Source: CAD feature listing. Evaluate the final solid. Frame: model axes, mm. A direction names the side the tool comes from. Give positions to 0.01 mm unless a question says otherwise; leave off trailing zeros. Order: outer loops, then holes, each group sorted by start corner. A loop starts at its lowest first (then second) coordinate and runs counter-clockwise, first axis right, second up.
```python
from build123d import *

# Parameters (mm, degrees)
BOSS_EXTRUDE1_DEPTH = 6.35
CUT_EXTRUDE1_DEPTH  = 212.713804804
SKETCH5_W           = 12.7
SKETCH5_H           = 30
CUT_EXTRUDE3_DEPTH  = 212.713804804


with BuildPart() as part:
    # Sketch2 → Boss-Extrude1 (new body)
    with BuildSketch(Plane(origin=(0, 0, 0), x_dir=(1, 0, 0), z_dir=(0, 1, 0))):
        with BuildLine():
            Line((-2.579558011, -38.687016575), (16.470441989, -38.687016575))
            Line((16.470441989, -38.687016575), (16.470441989, 20.312983425))
            Line((16.470441989, 20.312983425), (22.470441989, 20.312983425))
            ThreePointArc((22.470441989, 20.312983425), (23.17754877, 20.605876644), (23.470441989, 21.312983425))
            Line((23.470441989, 21.312983425), (23.470441989, 69.312983425))
            ThreePointArc((23.470441989, 69.312983425), (23.17754877, 70.020090207), (22.470441989, 70.312983425))
            Line((22.470441989, 70.312983425), (16.470441989, 70.312983425))
            Line((16.470441989, 70.312983425), (16.470441989, 130.312983425))
            Line((16.470441989, 130.312983425), (22.470441989, 130.312983425))
            ThreePointArc((22.470441989, 130.312983425), (23.17754877, 130.605876644), (23.470441989, 131.312983425))
            Line((23.470441989, 131.312983425), (23.470441989, 179.312983425))
            ThreePointArc((23.470441989, 179.312983425), (23.17754877, 180.020090207), (22.470441989, 180.312983425))
            Line((22.470441989, 180.312983425), (16.470441989, 180.312983425))
            Line((16.470441989, 180.312983425), (16.470441989, 210.312983425))
            Line((16.470441989, 210.312983425), (-2.579558011, 210.312983425))
            Line((-2.579558011, 210.312983425), (-2.579558011, -38.687016575))
        make_face()
    extrude(amount=BOSS_EXTRUDE1_DEPTH)

    # Sketch3 → Cut-Extrude1 (cut, through all)
    with BuildSketch(Plane(origin=(0, 6.35, 0), x_dir=(1, 0, 0), z_dir=(0, 1, 0))):
        with BuildLine():
            Line((16.470441989, 61.312983425), (4.470441989, 61.312983425))
            ThreePointArc((4.470441989, 61.312983425), (3.056228427, 61.898769863), (2.470441989, 63.312983425))
            Line((2.470441989, 63.312983425), (2.470441989, 89.312983425))
            ThreePointArc((2.470441989, 89.312983425), (3.056228427, 90.727196988), (4.470441989, 91.312983425))
            Line((4.470441989, 91.312983425), (16.470441989, 91.312983425))
            Line((16.470441989, 91.312983425), (16.470441989, 61.312983425))
        make_face()
    extrude(amount=-CUT_EXTRUDE1_DEPTH, mode=Mode.SUBTRACT)

    # Sketch5 → Cut-Extrude3 (cut, through all)
    with BuildSketch(Plane.XZ):
        with Locations((10.120441989, -116.312983425)):
            Rectangle(SKETCH5_W, SKETCH5_H)
    extrude(amount=-CUT_EXTRUDE3_DEPTH, mode=Mode.SUBTRACT)


solid = part.part
```
1) Draft query along Z for faces 4 (the flat face through (19, 3, -20.313)), 5 (the flat face through (16.47, 3, 10)), 6 (the flat face through (16.47, 3, -66)). Return one class per face: +Z half, -Z half, draft (parallel to the pull), parting line (faces both ways), or undercut.
Report:
face 4: +Z half
face 5: draft
face 6: undercut
2) Material intervals for L1, parallel to Z at x = 8.25, y = 2.5; L2, parallel to Z at x = 21.5, y = 3; L3, parallel to Z at x = 3.5, y = 5, sorted ascending.
Report:
L1: z = -210.31 to -131.31, -101.31 to -91.31, -61.31 to 38.69
L2: z = -180.31 to -130.31, -70.31 to -20.31
L3: z = -210.31 to -91.06, -61.56 to 38.69
3) Section query B-B, the plane y = 4.75. Return the cut outline in (x, z), and give its area (3 significant figures).
Report:
outline: (-2.58, -210.31) - (16.47, -210.31) - (16.47, -180.31) - (22.47, -180.31) arc R1 ccw to (23.47, -179.31) - (23.47, -131.31) arc R1 ccw to (22.47, -130.31) - (16.47, -130.31) - (16.47, -131.31) - (3.77, -131.31) - (3.77, -101.31) - (16.47, -101.31) - (16.47, -91.31) - (4.47, -91.31) arc R2 cw to (2.47, -89.31) - (2.47, -63.31) arc R2 cw to (4.47, -61.31) - (16.47, -61.31) - (16.47, -70.31) - (22.47, -70.31) arc R1 ccw to (23.47, -69.31) - (23.47, -21.31) arc R1 ccw to (22.47, -20.31) - (16.47, -20.31) - (16.47, 38.69) - (-2.58, 38.69) - close
area: 4,640 mm2
4) Reachability of faces 1 (the flat face through (16.47, 3, -96)), 2 (the flat face through (10, 3, -131.313)), 3 (the flat face through (16.47, 3, -195)) from +Z, -Z, +X, -X, +Y, -Y: full face, straight path, thin tool, end or side. Return the list, or none.
Report:
face 1: +X, +Y, -Y
face 2: +Y, -Y
face 3: -Z, +X, +Y, -Y
5) Section query C-C, the plane z = -105. Return the cut outline in (x, y).
Report:
outline: (-2.58, 0) - (3.77, 0) - (3.77, 6.35) - (-2.58, 6.35) - close
6) Pin query (flat end, axial travel): pin 1 (1.9 mm diameter, centred on y = 3, z = -188, fed in from +X); pin 2 (1.8 mm diameter, centred on x = 18.5, y = 2, fed in from -Z); pin 3 (3 mm diameter, centred on y = 4.5, z = -119.5, fed in from +X). Return the tip coordinate at first contact, or that it passes through.
Report:
pin 1: stops at x = 16.47
pin 2: stops at z = -180.31
pin 3: stops at x = 3.77
7) Section query A-A, the plane x = 20.25. Return the cut outline in (y, z), and give its area (3 significant figures).
Report:
outline: (0, -180.31) - (6.35, -180.31) - (6.35, -130.31) - (0, -130.31) - close; (0, -70.31) - (6.35, -70.31) - (6.35, -20.31) - (0, -20.31) - close
area: 635 mm2
